from build123d import *

# Parameters (mm, degrees)
SKETCH1_W           = 40
SKETCH1_H           = 59.46
SKETCH1_W_2         = 70
SKETCH1_H_2         = 20
BOSS_EXTRUDE1_DEPTH = 30


with BuildPart() as part:
    # Sketch1 → Boss-Extrude1 (new body)
    with BuildSketch(Plane.XY):
        with Locations((0, 39.73)):
            Rectangle(SKETCH1_W, SKETCH1_H)
        Rectangle(SKETCH1_W_2, SKETCH1_H_2)
    extrude(amount=BOSS_EXTRUDE1_DEPTH)


solid = part.part
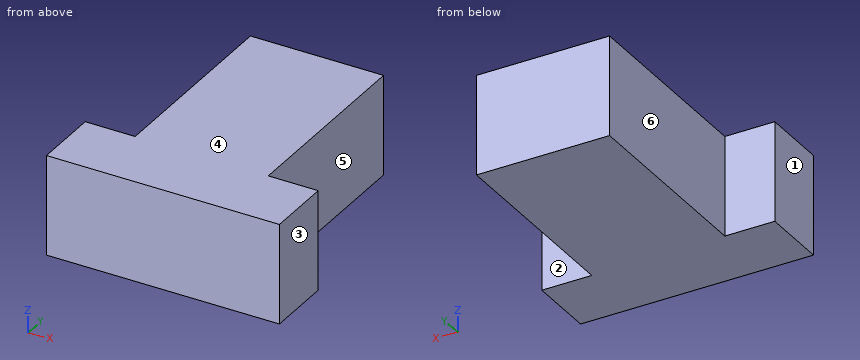
Here's how the part is built. I have some questions about the finished solid (model axes, mm). Face numbers are marked on the shaded views. A direction names the side the tool comes from. Round coordinates to 2 decimals unless told otherwise and drop trailing zeros. Write each loop counter-clockwise with the first axis right and the second up, starting at its lowest first coordinate (ties: lowest second). Pieces come first, ordered by that corner, then holes. Notation, with made-up numbers: (-40, 66) -> (0, 66) arc R11 ccw to (0, 73) -> close; hole circle Ø3 at (70, -20.75). An arc over 180 degrees is marked (long way). One line per item, written item: value.
1) Suppose I cut it at B-B on y = 41. List the corners of the cut face in (x, z) for me, plus the area to 3 significant figures.
Filled sheet:
outline: (-20, 0) -> (20, 0) -> (20, 30) -> (-20, 30) -> close
area: 1,200 mm2
2) We'd pull the mould along X, two halves only. Please class the marked faces 1, 2 and 3: released by +X, released by -X, zero draft, split by the parting line, or undercut.
Filled sheet:
face 1: released by -X
face 2: zero draft
face 3: released by +X
3) I'm going to push flat-ended pins straight in: pin 1 Ø15 at (y, z) = (41, 15) entering from +X; pin 2 Ø7.5 at (x, z) = (-24.5, 20) entering from +Y; pin 3 Ø1.5 at (x, y) = (1, 56.5) entering from -Z. Where does each tip first touch, or does it pass through?
Filled sheet:
pin 1: stops at x = 20
pin 2: stops at y = 10
pin 3: stops at z = 0
4) If I drill on line 1 (X direction, y = 49.5, z = 4.75); line 2 (Y direction, x = -26, z = 5.25), over which ranges is the centre line in solid material (lowest first)? Write a range as [from, to].
Filled sheet:
line 1: x = [-20, 20]
line 2: y = [-10, 10]
5) For the marked faces 4, 5 and 6, which set-ups out of +Z, -Z, +X, -X, +Y, -Y let a thin tool reach every point of the face, with its end or its side?
Filled sheet:
face 4: +Z, +X, -X, +Y, -Y
face 5: +Z, -Z, +X, +Y
face 6: +Z, -Z, -X, +Y
6) Suppose I cut it at C-C on x = -29.5. List the corners of the cut face in (y, z) for me, plus the area to 3 significant figures.
Filled sheet:
outline: (-10, 0) -> (10, 0) -> (10, 30) -> (-10, 30) -> close
area: 600 mm2
7) Suppose I cut it at A-A on z = 17.75. List the corners of the cut face in (x, y) for me, plus the area to 3 significant figures.
Filled sheet:
outline: (-35, -10) -> (35, -10) -> (35, 10) -> (20, 10) -> (20, 69.46) -> (-20, 69.46) -> (-20, 10) -> (-35, 10) -> close
area: 3,780 mm2
